CAD build for the part. Positions are in the model's coordinates, mm. Face numbers are marked on the shaded views. A direction names the side the tool comes from. Round coordinates to 2 decimals unless told otherwise and drop trailing zeros. Loops run counter-clockwise (first coordinate to the right, second up) from the corner with the lowest first, then second, coordinate; pieces in that order, holes last.
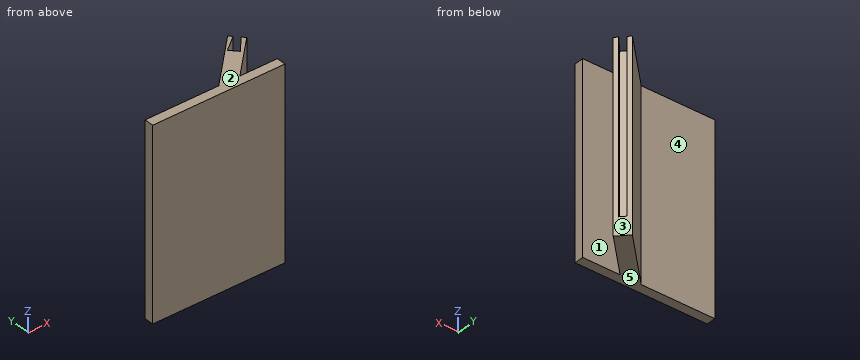
Autodesk Inventor part; units mm, degrees
ref_plane "YZ Plane" through (0, 0, 0) normal (1, 0, 0) x (0, 1, 0)
ref_plane "XZ Plane" through (0, 0, 0) normal (0, 1, 0) x (-1, 0, 0)
ref_plane "XY Plane" through (0, 0, 0) normal (0, 0, 1) x (1, 0, 0)
sketch "Sketch1" plane through (0, 0, 0) normal (0, 0, 1) x (1, 0, 0)
  line L0 (44.9013, -57.6013) -> (44.9013, -83.0013) construction
  line L1 (-44.9013, -83.0013) -> (44.9013, -83.0013)
  line L2 (-44.9013, -83.0013) -> (-44.9013, -89.3513)
  line L3 (44.9013, -83.0013) -> (44.9013, -89.3513)
  line L4 (44.9013, -83.0013) -> (51.2513, -83.0013) construction
  line L5 (-44.9013, -89.3513) -> (44.9013, -89.3513)
  line L6 (44.9013, -57.6013) -> (19.5013, -83.0013)
  line L7 (44.9013, -57.6013) -> (80.8223, -57.6013) construction
  line L8 (44.9013, -57.6013) -> (37.9664, -50.1761) construction
  line L9 (37.9664, -50.1761) -> (5.1412, -83.0013)
  line L10 (37.9664, -50.1761) -> (84.3883, -50.1761) construction
  line L11 (37.9664, -50.1761) -> (44.9013, -57.6013)
  dimension "d4" = 25.4
  dimension "d7" = 6.35
  dimension "d8" = 90
  dimension "d9" = 135
  dimension "d10" = 10.16
  dimension "d11" = 135
extrude "Extrusion1" add sketch "Sketch1" against normal blind 127
sketch "Sketch5" plane through (0, 0, 0) normal (0, 0, 1) x (1, 0, 0)
  line L0 (39.9602, -52.3108) -> (42.9075, -55.4665)
  line L1 (44.9013, -57.6013) -> (37.9664, -50.1761)
  line L2 (29.4406, -60.398) -> (34.1216, -65.41)
  line L3 (41.4339, -53.8887) -> (31.7811, -62.904) construction
  line L4 (29.4406, -60.398) -> (39.9602, -52.3108)
  line L5 (34.1216, -65.41) -> (42.9075, -55.4665)
  point P0 (0, 0)
  dimension "d28" = 4.318
  dimension "d29" = 6.858
  dimension "d30" = 13.208
extrude "Extrusion5" cut sketch "Sketch5" against normal blind 114.808
properties part number "proto_1_base"
Item 1: Cut at C-C, the plane x = -2.5. Give the cut face in (y, z).
Answers follow:
outline: (-89.35, -127) - (-83, -127) - (-83, 0) - (-89.35, 0) - close
Item 2: Cut at D-D, the plane y = -71. Give the cut face in (x, z), plus the area to 3 significant figures.
Answers follow:
outline: (17.14, -127) - (31.5, -127) - (31.5, 0) - (17.14, 0) - close
area: 1,820 mm2
Item 3: Flat gauge pins, fed straight in: P1, Ø5, axis at x = -6, z = -97.5, coming from the +Y side; P2, Ø4, axis at x = 34.5, y = -59.5, coming from the +Z side; P3, Ø6, axis at x = 12.5, z = -28, coming from the +Y side. Where does each tip first touch, or does it go through?
Answers follow:
P1: stops at y = -83
P2: stops at z = -114.81
P3: stops at y = -72.64
Item 4: Two-plate mould, pull along Y, no slides. Class the marked faces 1, 2 and 3: released by +Y, released by -Y, zero draft, split by the parting line, or undercut.
Answers follow:
face 1: undercut
face 2: zero draft
face 3: released by +Y
Item 5: Cut at B-B, the plane z = -21. Give the cut face in (x, y), plus the area to 4 significant figures.
Answers follow:
outline: (-44.9, -89.35) - (44.9, -89.35) - (44.9, -83) - (19.5, -83) - (44.9, -57.6) - (42.91, -55.47) - (34.12, -65.41) - (29.44, -60.4) - (39.96, -52.31) - (37.97, -50.18) - (5.14, -83) - (-44.9, -83) - close
area: 914.5 mm2
Item 6: Probe line 1 (Y direction, x = -34.5, z = -39); line 2 (Y direction, x = 27.5, z = -8.5); line 3 (X direction, y = -57.5, z = -72.5). List the from-to ranges inside material, lowest first.
Answers follow:
line 1: y = -89.35 to -83
line 2: y = -89.35 to -83, -75 to -60.64
line 3: x = 30.64 to 33.21, 41.11 to 44.81
Item 7: Cut at A-A, the plane x = 23.5. Give the cut face in (y, z).
Answers follow:
outline: (-89.35, -127) - (-83, -127) - (-83, 0) - (-89.35, 0) - close; (-79, -127) - (-64.64, -127) - (-64.64, 0) - (-79, 0) - close
Item 8: 3-axis set-ups, long thin cutter, end or side, ignore diameter. For the marked faces 4 and 5: which of +Z, -Z, +X, -X, +Y, -Y reach the whole face in a straight line?
Answers follow:
face 4: +Z, -Z, -X, +Y
face 5: -Z, +X, -X, +Y, -Y
